Model file for the job. Use its own axes, mm. Face numbers are marked on the shaded views. Round coordinates to 2 decimals unless told otherwise and drop trailing zeros. Write each loop counter-clockwise with the first axis right and the second up, starting at its lowest first coordinate (ties: lowest second). Pieces come first, ordered by that corner, then holes.
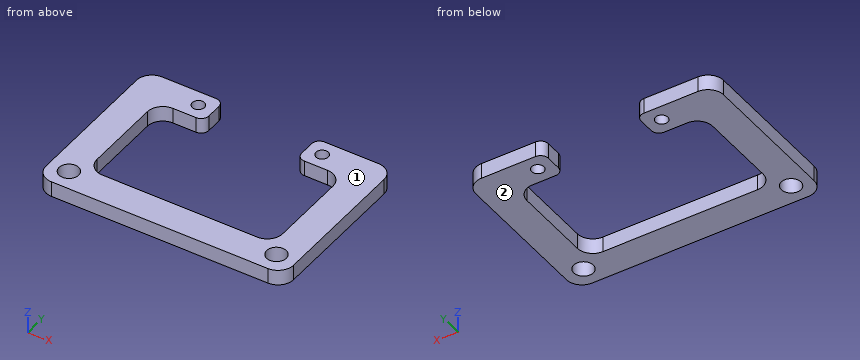
```python
from build123d import *

# Parameters (mm, degrees)
SKETCH1_R           = 6.35
SKETCH1_R_2         = 4
BOSS_EXTRUDE1_DEPTH = 5
FILLET1_R           = 10
FILLET2_R           = 5


with BuildPart() as part:
    # Sketch1 → Boss-Extrude1 (new, symmetric)
    with BuildSketch(Plane.XY):
        with BuildLine():
            Line((0, 20), (0, 0))
            Line((0, 0), (70, 0))
            ThreePointArc((70, 0), (77.071067812, 2.928932188), (80, 10))
            Line((80, 10), (80, 110))
            Line((80, 110), (30, 110))
            Line((30, 110), (30, 90))
            Line((30, 90), (60, 90))
            Line((60, 90), (60, 30))
            ThreePointArc((60, 30), (57.071067812, 22.928932188), (50, 20))
            Line((50, 20), (0, 20))
        make_face()
        with Locations((67.071067812, 12.928932188)):
            Circle(SKETCH1_R, mode=Mode.SUBTRACT)
        with Locations((40, 100)):
            Circle(SKETCH1_R_2, mode=Mode.SUBTRACT)
    boss_extrude1 = extrude(amount=BOSS_EXTRUDE1_DEPTH, both=True)

    # Mirror1: Boss-Extrude1 across plane
    add(boss_extrude1.mirror(Plane(origin=(0, 0, -5), x_dir=(0, 0, 1), z_dir=(-1, 0, 0))))

    # Fillet1
    fillet1_edges = [part.edges().sort_by_distance(p)[0] for p in [
        (60, 90, 0),
        (80, 110, 0),
        (-80, 110, 0),
        (-60, 90, 0),
    ]]
    fillet(fillet1_edges, radius=FILLET1_R)

    # Fillet2
    fillet2_edges = [part.edges().sort_by_distance(p)[0] for p in [
        (30, 90, 0),
        (30, 110, 0),
        (-30, 110, 0),
        (-30, 90, 0),
    ]]
    fillet(fillet2_edges, radius=FILLET2_R)


solid = part.part
```
1) Cut at A-A on x = 40. List the corners of the cut face in (y, z).
2) Flat gauge pins, fed straight in: pin 1 Ø7 at (x, y) = (-40, 100) entering from -Z; pin 2 Ø3 at (x, z) = (-14.5, -0.5) entering from +Y. Where does each tip first touch, or does it go through?
3) Pull direction Z, two halves, no side cores. Call the marked faces 1 and 2: released by +Z, released by -Z, zero draft, split by the parting line, or undercut.
4) Cut at C-C on z = -2.25. List the corners of the cut face in (x, y), and give its area (3 significant figures).
5) Cut at D-D on x = -54. List the corners of the cut face in (y, z), and give its area (3 significant figures).
6) Wall check: probe 1 along Y at (x, z) = (40, -2.5); probe 2 along X at (y, z) = (18, 3.5); probe 3 along X at (y, z) = (17, -3). Give the ranges that are in metal, low to high.
7) Cut at B-B on y = 44. List the corners of the cut face in (x, z).
Result sheet:
1. outline: (0, -5) - (20, -5) - (20, 5) - (0, 5) - close; (90, -5) - (96, -5) - (96, 5) - (90, 5) - close; (104, -5) - (110, -5) - (110, 5) - (104, 5) - close
2. pin 1: passes through
2. pin 2: stops at y = 20
3. face 1: released by +Z
3. face 2: released by -Z
4. outline: (-80, 10) arc R10 ccw to (-70, 0) - (70, 0) arc R10 ccw to (80, 10) - (80, 100) arc R10 ccw to (70, 110) - (35, 110) arc R5 ccw to (30, 105) - (30, 95) arc R5 ccw to (35, 90) - (50, 90) arc R10 cw to (60, 80) - (60, 30) arc R10 cw to (50, 20) - (-50, 20) arc R10 cw to (-60, 30) - (-60, 80) arc R10 cw to (-50, 90) - (-35, 90) arc R5 ccw to (-30, 95) - (-30, 105) arc R5 ccw to (-35, 110) - (-70, 110) arc R10 ccw to (-80, 100) - close; hole circle Ø12.7 at (-67.07, 12.93); hole circle Ø8 at (-40, 100); hole circle Ø8 at (40, 100); hole circle Ø12.7 at (67.07, 12.93)
4. area: 7,620 mm2
5. outline: (0, -5) - (20.83, -5) - (20.83, 5) - (0, 5) - close; (89.17, -5) - (110, -5) - (110, 5) - (89.17, 5) - close
5. area: 417 mm2
6. probe 1: y = 0 to 20, 90 to 96, 104 to 110
6. probe 2: x = -80 to -70.89, -63.25 to 63.25, 70.89 to 80
6. probe 3: x = -80 to -71.94, -62.2 to 62.2, 71.94 to 80
7. outline: (-80, -5) - (-60, -5) - (-60, 5) - (-80, 5) - close; (60, -5) - (80, -5) - (80, 5) - (60, 5) - close
